CAD build for the part. Positions are in the model's coordinates, mm. A direction names the side the tool comes from. Give positions to 0.01 mm unless a question says otherwise; leave off trailing zeros. Write each loop counter-clockwise with the first axis right and the second up, starting at its lowest first coordinate (ties: lowest second). Pieces come first, ordered by that corner, then holes. Notation, with made-up numbers: (-27, 50) -> (27, 50) arc R28 ccw to (27, 89) -> close; hole circle Ø1 at (-13, 47). An arc over 180 degrees is marked (long way). Answer as a JSON object with one key per item and string values.
```python
from build123d import *

# Parameters (mm, degrees)
F1_DEPTH = 8.89
F2_R     = 9.525
F3_DEPTH = 9.144
F4_R     = 11.176
F5_DEPTH = 7.112


with BuildPart() as f1:
    # F0 (on Front) → F1 (new body)
    with BuildSketch(Plane.XZ):
        with BuildLine():
            Line((33.02, 7.69326929), (33.02, -7.69326929))
            Line((33.02, -7.69326929), (19.8643469326, -7.69326929))
            ThreePointArc((19.8643469326, -7.69326929), (37.0053134916, -14.7096864812), (48.26, 0))
            ThreePointArc((48.26, 0), (37.0053134916, 14.7096864812), (19.8643469326, 7.69326929))
            Line((19.8643469326, 7.69326929), (33.02, 7.69326929))
        make_face()
        with BuildLine():
            Line((19.8643469326, -7.69326929), (33.02, -7.69326929))
            Line((33.02, -7.69326929), (33.02, 7.69326929))
            Line((33.02, 7.69326929), (19.8643469326, 7.69326929))
            ThreePointArc((19.8643469326, 7.69326929), (17.78, 0), (19.8643469326, -7.69326929))
        make_face()
        with BuildLine():
            Line((13.1556530674, -7.69326929), (19.8643469326, -7.69326929))
            ThreePointArc((19.8643469326, -7.69326929), (17.78, 0), (19.8643469326, 7.69326929))
            Line((19.8643469326, 7.69326929), (13.1556530674, 7.69326929))
            ThreePointArc((13.1556530674, 7.69326929), (14.7096864812, 3.9853134916), (15.24, 0))
            ThreePointArc((15.24, 0), (14.7096864812, -3.9853134916), (13.1556530674, -7.69326929))
        make_face()
        with BuildLine():
            ThreePointArc((-13.1556530674, -7.69326929), (0, -15.24), (13.1556530674, -7.69326929))
            Line((13.1556530674, -7.69326929), (-13.1556530674, -7.69326929))
        make_face()
        with BuildLine():
            Line((-13.1556530674, -7.69326929), (13.1556530674, -7.69326929))
            ThreePointArc((13.1556530674, -7.69326929), (14.7096864812, -3.9853134916), (15.24, 0))
            ThreePointArc((15.24, 0), (14.7096864812, 3.9853134916), (13.1556530674, 7.69326929))
            Line((13.1556530674, 7.69326929), (-13.1556530674, 7.69326929))
            ThreePointArc((-13.1556530674, 7.69326929), (-15.24, 0), (-13.1556530674, -7.69326929))
        make_face()
        with BuildLine():
            Line((-19.8643469326, -7.69326929), (-13.1556530674, -7.69326929))
            ThreePointArc((-13.1556530674, -7.69326929), (-15.24, 0), (-13.1556530674, 7.69326929))
            Line((-13.1556530674, 7.69326929), (-19.8643469326, 7.69326929))
            ThreePointArc((-19.8643469326, 7.69326929), (-18.3103135188, 3.9853134916), (-17.78, 0))
            ThreePointArc((-17.78, 0), (-18.3103135188, -3.9853134916), (-19.8643469326, -7.69326929))
        make_face()
        with BuildLine():
            Line((-13.1556530674, 7.69326929), (13.1556530674, 7.69326929))
            ThreePointArc((13.1556530674, 7.69326929), (0, 15.24), (-13.1556530674, 7.69326929))
        make_face()
        with BuildLine():
            ThreePointArc((-19.8643469326, 7.69326929), (-48.26, 0), (-19.8643469326, -7.69326929))
            Line((-19.8643469326, -7.69326929), (-33.02, -7.69326929))
            Line((-33.02, -7.69326929), (-33.02, 7.69326929))
            Line((-33.02, 7.69326929), (-19.8643469326, 7.69326929))
        make_face()
        with BuildLine():
            Line((-33.02, -7.69326929), (-19.8643469326, -7.69326929))
            ThreePointArc((-19.8643469326, -7.69326929), (-18.3103135188, -3.9853134916), (-17.78, 0))
            ThreePointArc((-17.78, 0), (-18.3103135188, 3.9853134916), (-19.8643469326, 7.69326929))
            Line((-19.8643469326, 7.69326929), (-33.02, 7.69326929))
            Line((-33.02, 7.69326929), (-33.02, -7.69326929))
        make_face()
    extrude(amount=F1_DEPTH)

    # F2 (on face) → F3 (cut)
    with BuildSketch(Plane.XZ.offset(8.89)):
        Circle(F2_R)
        with Locations((33.02, 0)):
            Circle(F2_R)
        with Locations((-33.02, 0)):
            Circle(F2_R)
    extrude(amount=-F3_DEPTH, mode=Mode.SUBTRACT)

    # F4 (on face) → F5 (cut)
    with BuildSketch(Plane.XZ.offset(8.89)):
        Circle(F4_R)
        with Locations((-33.02, 0)):
            Circle(F4_R)
        with Locations((33.02, 0)):
            Circle(F4_R)
    extrude(amount=-F5_DEPTH, mode=Mode.SUBTRACT)


solid = f1.part
```
1) Slice it at C-C (z = -6). List the corners of the cut face in (x, y).
Model answer:
{"outline": "(-47.03, -8.89) -> (-42.45, -8.89) -> (-42.45, -1.78) -> (-40.42, -1.78) -> (-40.42, 0) -> (-47.03, 0) -> close; (-25.62, -1.78) -> (-23.59, -1.78) -> (-23.59, -8.89) -> (-9.43, -8.89) -> (-9.43, -1.78) -> (-7.4, -1.78) -> (-7.4, 0) -> (-25.62, 0) -> close; (7.4, -1.78) -> (9.43, -1.78) -> (9.43, -8.89) -> (23.59, -8.89) -> (23.59, -1.78) -> (25.62, -1.78) -> (25.62, 0) -> (7.4, 0) -> close; (40.42, -1.78) -> (42.45, -1.78) -> (42.45, -8.89) -> (47.03, -8.89) -> (47.03, 0) -> (40.42, 0) -> close"}
2) Slice it at A-A (y = -7.5). List the corners of the cut face in (x, z).
Model answer:
{"outline": "(-19.86, -7.69) -> (-13.16, -7.69) arc R15.24 ccw to (13.16, -7.69) -> (19.86, -7.69) arc R15.24 ccw (long way) to (19.86, 7.69) -> (13.16, 7.69) arc R15.24 ccw to (-13.16, 7.69) -> (-19.86, 7.69) arc R15.24 ccw (long way) to start; hole circle Ø22.35 at (-33.02, 0); hole circle Ø22.35 at (0, 0); hole circle Ø22.35 at (33.02, 0)"}
3) Slice it at B-B (x = -33.02). List the corners of the cut face in (y, z) (3 decimals).
Model answer:
{"outline": "(-8.89, -15.24) -> (0, -15.24) -> (0, -9.525) -> (-1.778, -9.525) -> (-1.778, -11.176) -> (-8.89, -11.176) -> close; (-8.89, 11.176) -> (-1.778, 11.176) -> (-1.778, 9.525) -> (0, 9.525) -> (0, 15.24) -> (-8.89, 15.24) -> close"}
4) Slice it at D-D (x = 36.5). List the corners of the cut face in (y, z), then the cut area to 3 significant figures.
Model answer:
{"outline": "(-8.89, -14.84) -> (0, -14.84) -> (0, -8.87) -> (-1.78, -8.87) -> (-1.78, -10.62) -> (-8.89, -10.62) -> close; (-8.89, 10.62) -> (-1.78, 10.62) -> (-1.78, 8.87) -> (0, 8.87) -> (0, 14.84) -> (-8.89, 14.84) -> close", "area": "81.2 mm2"}
5) Pin check, flat tips, straight feed: pin 1 (5 mm diameter, centred on y = -1, z = -11, fed in from +X); pin 2 (2 mm diameter, centred on x = -16.5, y = -5.5, fed in from +Z); pin 3 (11.5 mm diameter, centred on x = 33.02, z = 0, fed in from -Y); pin 4 (1.5 mm diameter, centred on x = -7, y = -5, fed in from +Z). Stop position of each tip, or through.
Model answer:
{"pin 1": "stops at x = 45.67", "pin 2": "stops at z = 7.69", "pin 3": "passes through", "pin 4": "stops at z = 13.9"}
6) Wall check: probe 1 along X at (y, z) = (-7.5, 2.5); probe 2 along X at (y, z) = (-3.5, 13); probe 3 along X at (y, z) = (-5.5, -4). Give the ranges that are in metal, low to high.
Model answer:
{"probe 1": "x = -48.05 to -43.91, -22.13 to -10.89, 10.89 to 22.13, 43.91 to 48.05", "probe 2": "x = -40.97 to -25.07, -7.95 to 7.95, 25.07 to 40.97", "probe 3": "x = -47.73 to -43.46, -22.58 to -10.44, 10.44 to 22.58, 43.46 to 47.73"}
7) 3-axis set-ups, long thin cutter, end or side, ignore diameter. For faces 1 (the flat face through (-17, -4, -7.693)), 2 (the flat face through (17, -4, 7.693)), 3 (the flat face through (-11.4, -8.89, 0.2)), 4 (the flat face through (42.1, -1.778, 3.4)), 5 (the cylindrical face through (-48.25, -4.38, 0.56)): which of +Z, -Z, +X, -X, +Y, -Y reach the whole face in a straight line?
Model answer:
{"face 1": "-Z, +Y, -Y", "face 2": "+Z, +Y, -Y", "face 3": "+Z, -Z, +X, -X, -Y", "face 4": "-Y", "face 5": "+Y, -Y"}
8) Mould opens along Z. For faces 6 (the flat face through (-16, -4, 7.693)), 7 (the flat face through (9.1, -1.778, 3.4)), 8 (the cylindrical face through (-0.22, -4.38, -15.24)) say: released by +Z, released by -Z, zero draft, split by the parting line, or undercut.
Model answer:
{"face 6": "released by +Z", "face 7": "undercut", "face 8": "released by -Z"}
